Can you work these out from the model? Positions are in its coordinate system, mm. A direction names the side the tool comes from. Round coordinates to 2 decimals unless told otherwise and drop trailing zeros. Order: outer loops, then holes, each group sorted by start corner. A loop starts at its lowest first (then second) coordinate and runs counter-clockwise, first axis right, second up. Notation, with made-up numbers: (-28, 9) - (19, 9) arc R18 ccw to (19, 42) - close; hole circle Ø4 at (80.25, 70). An arc over 180 degrees is marked (long way). Write item = value, one per line.
from build123d import *

# Parameters (mm, degrees)
SKETCH1_R           = 101.6
SKETCH1_R_2         = 20
BOSS_EXTRUDE1_DEPTH = 50.8
SKETCH2_R           = 95.25
SKETCH2_R_2         = 25
CUT_EXTRUDE1_DEPTH  = 6.35
CUT_EXTRUDE2_START  = -6.35
SKETCH3_R           = 95.25
SKETCH3_R_2         = 25
CUT_EXTRUDE2_DEPTH  = 6.35


with BuildPart() as part:
    # Sketch1 → Boss-Extrude1 (new body)
    with BuildSketch(Plane(origin=(0, 0, 0), x_dir=(0, 0, -1), z_dir=(1, 0, 0))):
        Circle(SKETCH1_R)
        Circle(SKETCH1_R_2, mode=Mode.SUBTRACT)
    extrude(amount=BOSS_EXTRUDE1_DEPTH)

    # Sketch2 → Cut-Extrude1 (cut)
    with BuildSketch(Plane.ZY):
        Circle(SKETCH2_R)
        Circle(SKETCH2_R_2, mode=Mode.SUBTRACT)
    extrude(amount=-CUT_EXTRUDE1_DEPTH, mode=Mode.SUBTRACT)

    # Sketch3 → Cut-Extrude2 (cut)
    with BuildSketch(Plane(origin=(50.8, 0, 0), x_dir=(0, 0, -1), z_dir=(1, 0, 0)).offset(CUT_EXTRUDE2_START)):
        with Locations(Location((0, 0, 0), (0, 0, 180))):
            Circle(SKETCH3_R)
        with Locations(Location((0, 0, 0), (0, 0, 180))):
            Circle(SKETCH3_R_2, mode=Mode.SUBTRACT)
    extrude(amount=CUT_EXTRUDE2_DEPTH, mode=Mode.SUBTRACT)


solid = part.part
(1) On a 3-axis mill with a long thin cutter (end or side, diameter ignored), from which of +Z, -Z, +X, -X, +Y, -Y can I reach the whole of each face in a straight line? I mean faces 4 (the face through (6.35, -20, 20)), 5 (the face through (47.581, -7.509, 23.846)), 6 (the face through (50.8, 17, 11)). Say none if no direction works.
Computed:
face_4 = -X
face_5 = +X
face_6 = +Z, -Z, +X, +Y, -Y
(2) If we section it at D-D (y = 84): Write out the boundary of the cut face in (x, z), plus the area to 3 significant figures.
Computed:
outline = (0, -57.15) - (50.8, -57.15) - (50.8, -44.91) - (44.45, -44.91) - (44.45, 44.91) - (50.8, 44.91) - (50.8, 57.15) - (0, 57.15) - (0, 44.91) - (6.35, 44.91) - (6.35, -44.91) - (0, -44.91) - close
area = 4,670 mm^2
(3) Will these pins go through, and if not, where does the flat tip stop? P1, Ø3, axis at x = 27.5, y = 64, coming from the +Z side; P2, Ø1.5, axis at y = 58.5, z = -19, coming from the +X side; P3, Ø8, axis at y = -74, z = 53.5, coming from the +X side; P4, Ø10, axis at y = 20.5, z = 40, coming from the -X side.
Computed:
P1 = 80.1
P2 = 44.45
P3 = 50.8
P4 = 6.35
(4) If we section it at A-A (y = 0): Write out the boundary of the cut face in (x, z), plus the area to 3 significant figures.
Computed:
outline = (0, -101.6) - (50.8, -101.6) - (50.8, -95.25) - (44.45, -95.25) - (44.45, -25) - (50.8, -25) - (50.8, -20) - (0, -20) - (0, -25) - (6.35, -25) - (6.35, -95.25) - (0, -95.25) - close; (0, 20) - (50.8, 20) - (50.8, 25) - (44.45, 25) - (44.45, 95.25) - (50.8, 95.25) - (50.8, 101.6) - (0, 101.6) - (0, 95.25) - (6.35, 95.25) - (6.35, 25) - (0, 25) - close
area = 6,510 mm^2
(5) If I drill on line 1 (Y direction, x = 47.5, z = 0); line 2 (Z direction, x = 6, y = -20.5); line 3 (Z direction, x = 40, y = -6), over which ranges is the centre line in solid material (lowest first)? Write a range as from..to.
Computed:
line_1 = -101.6..-95.25, -25..-20, 20..25, 95.25..101.6
line_2 = -99.51..-93.02, -14.31..14.31, 93.02..99.51
line_3 = -101.42..-19.08, 19.08..101.42
(6) Thinking about a two-plate mould opening in Z: for faces 1 (the face through (0, -30, 91)), 2 (the face through (25.044, -99.184, 22.025)), 3 (the face through (25.044, -19.524, 4.336)), which applies, +Z half, -Z half, draft (parallel to the pull), parting line (faces both ways), or undercut?
Computed:
face_1 = draft
face_2 = parting line
face_3 = undercut
(7) If we section it at C-C (x = 23.5): Write out the boundary of the cut face in (y, z).
Computed:
outline = circle Ø203.2 at (0, 0); hole circle Ø40 at (0, 0)
